```python
from build123d import *

# Parameters (mm, degrees)
SKICA1_W                 = 7.5
SKICA1_H                 = 9
P_IDAT_VYSUNUT_M1_DEPTH  = 3.5
ZAOBLIT1_R               = 1
SKICA2_W                 = 1.5
SKICA2_H                 = 7
ODEBRAT_VYSUNUT_M1_DEPTH = 5


with BuildPart() as part:
    # Skica1 → Přidat vysunutím1 (new body)
    with BuildSketch(Plane.XY):
        Rectangle(SKICA1_W, SKICA1_H)
    extrude(amount=P_IDAT_VYSUNUT_M1_DEPTH)

    # Zaoblit1
    zaoblit1_edges = [part.edges().sort_by_distance(p)[0] for p in [
        (0, -4.5, 3.5),
        (0, -4.5, 0),
        (0, 4.5, 0),
        (0, 4.5, 3.5),
    ]]
    fillet(zaoblit1_edges, radius=ZAOBLIT1_R)

    # Skica2 → Odebrat vysunutím1 (cut)
    with BuildSketch(Plane(origin=(3.75, 0, 0), x_dir=(0, 0, -1), z_dir=(1, 0, 0))):
        with Locations((-1.75, 0)):
            Rectangle(SKICA2_W, SKICA2_H)
    extrude(amount=-ODEBRAT_VYSUNUT_M1_DEPTH, mode=Mode.SUBTRACT)


solid = part.part
```
For this review, take the finished solid that the model builds, in its own axes (mm). A direction names the side the tool comes from. Coordinates: 2 decimals unless noted, no trailing zeros. Loops run counter-clockwise (first coordinate to the right, second up) from the corner with the lowest first, then second, coordinate; pieces in that order, holes last. Notation, with made-up numbers: (-36.75, 7) - (2.25, 7) arc R9 cw to (2.25, 12) - close; hole circle Ø9 at (26, 55). An arc over 180 degrees is marked (long way). Use one line per item in the form item = value. Start each with the question number.
1) To check wall thickness, follow probe 1 along Z at (x, y) = (1.75, -0.75); probe 2 along Y at (x, z) = (2.75, 2.35); probe 3 along X at (y, z) = (-1, 1.5). State the ranges of each line that lie inside material, in increasing order. Write a range as from..to.
2) Take a section at D-D (z = 3.25). State the section outline as (x, y) points, plus the area to 3 significant figures.
3) Draft analysis for pull direction Z (two halves, no side actions). For faces 3 (the face through (0.053, 4.215, 0.301)), 4 (the face through (1, 0, 1)), 5 (the face through (0, 0, 3.5)), state which applies: released by +Z, released by -Z, zero draft, split by the parting line, or undercut.
4) Take a section at A-A (y = -2.25). State the section outline as (x, z) points, plus the area to 4 significant figures.
5) Take a section at C-C (z = 1.45). State the section outline as (x, y) points, plus the area to 3 significant figures.
6) For faces 1 (the face through (1, 3.5, 2)), 2 (the face through (-3.75, 0, 2)), list the 3-axis set-ups (+Z, -Z, +X, -X, +Y, -Y) from which the entire face can be reached by the end or side of a thin tool; tool diameter is ignored.
7) Take a section at B-B (x = -0.25). State the section outline as (y, z) points.
From the geometry:
q1.probe_1 = 0..1, 2.5..3.5
q1.probe_2 = -4.5..-3.5, 3.5..4.5
q1.probe_3 = -3.75..-1.25
q2.outline = (-3.75, -4.16) - (3.75, -4.16) - (3.75, 4.16) - (-3.75, 4.16) - close
q2.area = 62.4 mm2
q3.face_3 = released by -Z
q3.face_4 = undercut
q3.face_5 = released by +Z
q4.outline = (-3.75, 0) - (3.75, 0) - (3.75, 1) - (-1.25, 1) - (-1.25, 2.5) - (3.75, 2.5) - (3.75, 3.5) - (-3.75, 3.5) - close
q4.area = 18.75 mm2
q5.outline = (-3.75, -4.5) - (3.75, -4.5) - (3.75, -3.5) - (-1.25, -3.5) - (-1.25, 3.5) - (3.75, 3.5) - (3.75, 4.5) - (-3.75, 4.5) - close
q5.area = 32.5 mm2
q6.face_1 = +X
q6.face_2 = +Z, -Z, -X, +Y, -Y
q7.outline = (-4.5, 1) arc R1 ccw to (-3.5, 0) - (3.5, 0) arc R1 ccw to (4.5, 1) - (4.5, 2.5) arc R1 ccw to (3.5, 3.5) - (-3.5, 3.5) arc R1 ccw to (-4.5, 2.5) - close; hole (-3.5, 1) - (3.5, 1) - (3.5, 2.5) - (-3.5, 2.5) - close
